The figure shows three views and two pictorial views of one solid part (mm, origin at its lowest corner). Answer the questions. A direction names the side the tool comes from. Round coordinates to 2 decimals unless told otherwise and drop trailing zeros. Order: outer loops, then holes, each group sorted by start corner. A loop starts at its lowest first (then second) coordinate and runs counter-clockwise, first axis right, second up. Notation, with made-up numbers: (-19.75, 29) -> (22.25, 29) arc R29 cw to (22.25, 56) -> close; hole circle Ø10 at (-26.75, -14). An arc over 180 degrees is marked (long way). Return JSON: item names as keys, results as strings. Group by question number.
(1) Consider line 1 (Z direction, x = 9.25, y = 2.75); line 2 (X direction, y = 4, z = 3.75) (1 decimal); line 3 (Z direction, x = 14.75, y = 4.5) (1 decimal). Determine where each line is inside the solid, lowest interval first. Write a range as [from, to].
(2) The part is cut by section C-C (y = 5.5). Determine the outline of the cut face in (x, z).
(3) The part is cut by section B-B (y = 1.5). Count the separate pieces of the cut face and the enclosed holes in it, plus the area to 3 significant figures.
(4) Which of the six approach directions +Z, -Z, +X, -X, +Y, -Y give full straight-line access (tool end or side, diameter ignored) to the marked faces 1 and 2?
(5) Each of these flat-tipped pins is pushed along its axis until it touches: pin 1 (3 mm diameter, centred on x = 14, z = 13, fed in from +Y); pin 2 (3 mm diameter, centred on x = 13.5, y = 3.5, fed in from +Z); pin 3 (4 mm diameter, centred on y = 3, z = 3.5, fed in from -X) (1 decimal). Where does it stop, or does it pass through?
(6) Determine the mould class of the marked faces 3, 4 and 5 for opening direction Z: +Z half, -Z half, draft (parallel to the pull), parting line (faces both ways), or undercut.
(7) The part is cut by section A-A (x = 9.25). Determine the outline of the cut face in (y, z).
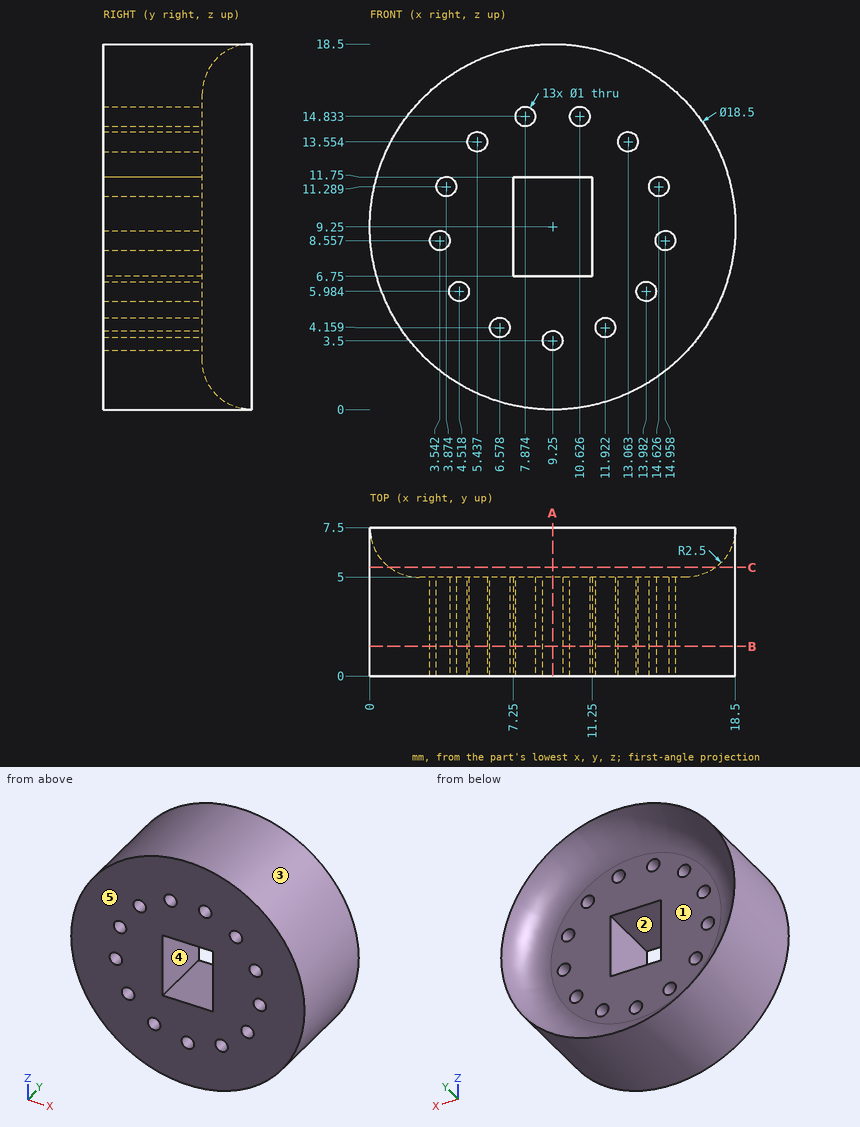
Answer below:
{
 "1": {"line 1": "z = [0, 3], [4, 6.75], [11.75, 18.5]", "line 2": "x = [1.8, 6.3], [6.9, 8.8], [9.7, 11.6], [12.2, 16.7]", "line 3": "z = [1.8, 8.1], [9, 10.8], [11.8, 16.7]"},
 "2": {"outline": "circle Ø18.5 at (9.25, 9.25); hole circle Ø16.5 at (9.25, 9.25)"},
 "3": {"separate pieces": "1", "enclosed holes": "14", "area": "239 mm²"},
 "4": {"face 1": "+Y", "face 2": "+Y, -Y"},
 "5": {"pin 1": "stops at y = 5.13", "pin 2": "stops at z = 18.08", "pin 3": "stops at x = 0.8"},
 "6": {"face 3": "parting line", "face 4": "undercut", "face 5": "draft"},
 "7": {"outline": "(0, 0) -> (7.5, 0) arc R2.5 cw to (5, 2.5) -> (5, 3) -> (0, 3) -> close; (0, 4) -> (5, 4) -> (5, 6.75) -> (0, 6.75) -> close; (0, 11.75) -> (5, 11.75) -> (5, 16) arc R2.5 cw to (7.5, 18.5) -> (0, 18.5) -> close"}
}
